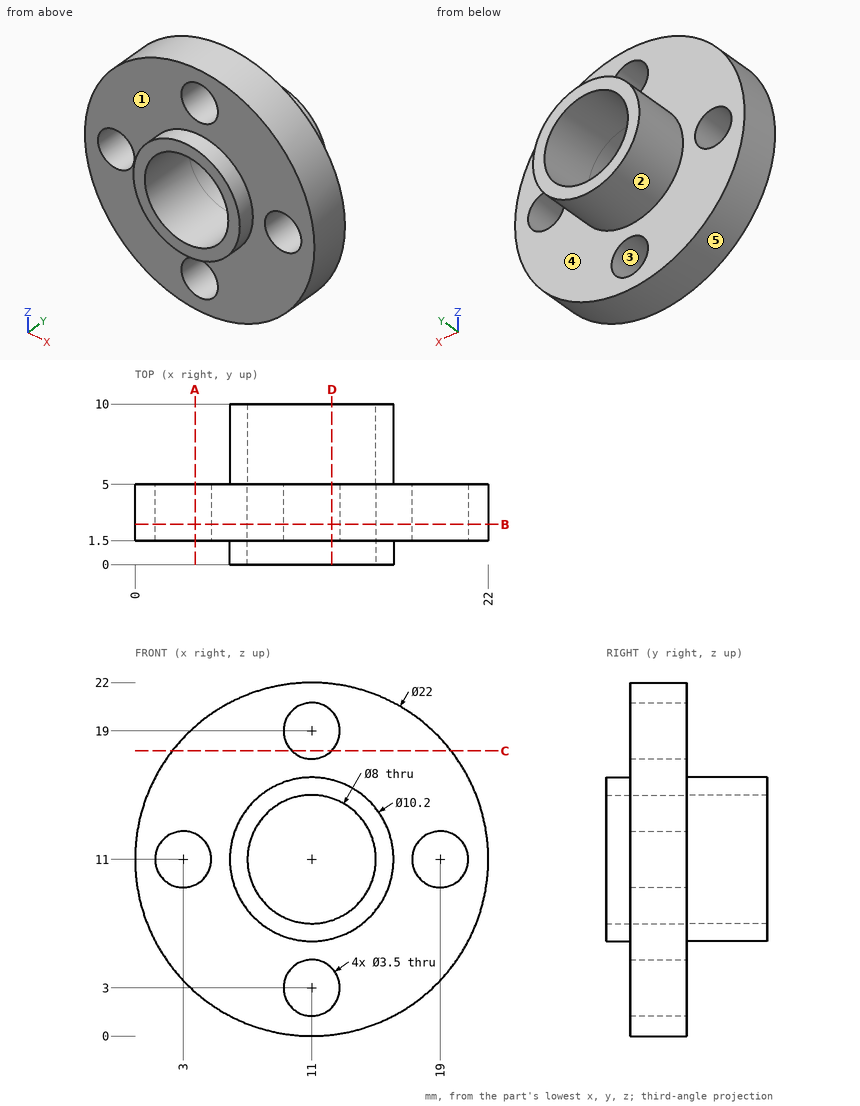
Geometry check sheet. Reference: drawing and pictorial views, mm from the part's lowest x, y, z. A direction names the side the tool comes from. Round coordinates to 2 decimals unless told otherwise and drop trailing zeros. Order: outer loops, then holes, each group sorted by start corner. A loop starts at its lowest first (then second) coordinate and runs counter-clockwise, first axis right, second up. Notation, with made-up numbers: M 15,78.5 L 62,78.5 A13 ccw 62,103.5 Z; hole C 79,-36.5 d5. An arc over 180 degrees is marked long. One line per item, written item: value. Start each with the question number.
1. Release check for a two-part mould opening along X. For the marked faces 1, 2 and 3 record: released by +X, released by -X, zero draft, split by the parting line, or undercut.
2. Access from +Z, -Z, +X, -X, +Y, -Y to the whole of each face (thin tool, end or side, straight path). Record for the marked faces 4 and 5.
3. Section check D-D on x = 12.25. Enter the section's corners in (y, z).
4. Section check C-C on z = 17.75. Enter the section's corners in (x, y), and give its area (3 significant figures).
5. Gauge pin test, flat ends, axial feed: P1, Ø1, axis at y = 8.5, z = 4, coming from the +X side; P2, Ø4, axis at x = 17, z = 9.5, coming from the -Y side; P3, Ø4.5, axis at x = 3, z = 11, coming from the +Y side; P4, Ø3, axis at y = 5.5, z = 17, coming from the -X side. Record the tip position at first contact, or that the pin passes through.
6. Section check A-A on x = 3.75. Enter the section's corners in (y, z).
7. Section check B-B on y = 2.5. Enter the section's corners in (x, z).
8. Scan lines: line 1 along Z through (x, y) = (11, 3.6); line 2 along X through (y, z) = (4.25, 12); line 3 along Y through (x, z) = (19.75, 16). Record each from-to range of solid material in increasing order.
Results found:
1. face 1: zero draft
1. face 2: split by the parting line
1. face 3: undercut
2. face 4: +Y
2. face 5: +Y, -Y
3. outline: M 0,6.06 L 1.5,6.06 L 1.5,4.22 L 5,4.22 L 5,6.06 L 10,6.06 L 10,7.2 L 0,7.2 Z; M 0,14.8 L 10,14.8 L 10,15.94 L 5,15.94 L 5,17.78 L 1.5,17.78 L 1.5,15.94 L 0,15.94 Z; M 1.5,0.07 L 5,0.07 L 5,1.78 L 1.5,1.78 Z; M 1.5,20.22 L 5,20.22 L 5,21.93 L 1.5,21.93 Z
4. outline: M 2.31,1.5 L 9.78,1.5 L 9.78,5 L 2.31,5 Z; M 12.22,1.5 L 19.69,1.5 L 19.69,5 L 12.22,5 Z
4. area: 52.2 mm^2
5. P1: through
5. P2: y = 0
5. P3: y = 5
5. P4: x = 1
6. outline: M 1.5,2.73 L 5,2.73 L 5,9.42 L 1.5,9.42 Z; M 1.5,12.58 L 5,12.58 L 5,19.27 L 1.5,19.27 Z
7. outline: C 11,11 d22; hole C 3,11 d3.5; hole C 11,11 d8; hole C 11,3 d3.5; hole C 11,19 d3.5; hole C 19,11 d3.5
8. line 1: 0 to 1.25, 4.75 to 7, 15 to 17.25, 20.75 to 22
8. line 2: 0.05 to 1.56, 4.44 to 7.13, 14.87 to 17.56, 20.44 to 21.95
8. line 3: 1.5 to 5
